The listing builds one solid part. Answer for the finished solid, in the listing's coordinates (mm). A direction names the side the tool comes from. Coordinates: 2 decimals unless noted, no trailing zeros. Order: outer loops, then holes, each group sorted by start corner. A loop starts at its lowest first (then second) coordinate and runs counter-clockwise, first axis right, second up. Notation, with made-up numbers: (43, 4) -> (91, 4) arc R22 ccw to (91, 16) -> close; hole circle Ø7 at (-20, 45). An arc over 180 degrees is marked (long way). Return JSON: item names as keys, results as strings.
```python
from build123d import *

# Parameters (mm, degrees)
REVOLVE_OF_12_NOM_W          = 584.2
REVOLVE_OF_12_NOM_H          = 20.193
F_6_NOM_OD_EXTRUDE_REACH     = 570.325
SKETCH2_R                    = 84.1375
F_6_NOM_ID_EXTRUDE_CUT_REACH = 570.325
F_6_NOM_ID_EXTRUDE_R         = 73.6473


with BuildPart() as part:
    # Revolve of 12 NOM → Revolve12 NOM (revolve)
    with BuildSketch(Plane.XY):
        with Locations((0, 151.8285)):
            Rectangle(REVOLVE_OF_12_NOM_W, REVOLVE_OF_12_NOM_H)
    revolve(axis=Axis((0, 0, 0), (1, 0, 0)))

    # Sketch2 → 6 NOM OD Extrude (add, up to next)
    with BuildSketch(Plane(origin=(0, 406.4, 0), x_dir=(1, 0, 0), z_dir=(0, 1, 0)), mode=Mode.PRIVATE) as f_6_nom_od_extrude_sk1:
        Circle(SKETCH2_R)
    f_6_nom_od_extrude_tool1 = extrude(f_6_nom_od_extrude_sk1.sketch, amount=-F_6_NOM_OD_EXTRUDE_REACH, mode=Mode.PRIVATE) - part.part
    add(f_6_nom_od_extrude_tool1.solids().sort_by_distance((0, 406.4, 0))[0])

    # 6 NOM ID Extrude → 6 NOM ID Extrude Cut (cut, up to next)
    with BuildSketch(Plane(origin=(0, 406.4, 0), x_dir=(1, 0, 0), z_dir=(0, 1, 0)), mode=Mode.PRIVATE) as f_6_nom_id_extrude_cut_sk1:
        Circle(F_6_NOM_ID_EXTRUDE_R)
    f_6_nom_id_extrude_cut_tool1 = extrude(f_6_nom_id_extrude_cut_sk1.sketch, amount=-F_6_NOM_ID_EXTRUDE_CUT_REACH, mode=Mode.PRIVATE) & part.part
    add(f_6_nom_id_extrude_cut_tool1.solids().sort_by_distance((0, 406.4, 0))[0], mode=Mode.SUBTRACT)


solid = part.part
```
Item 1: Find the intervals of material crossed by probe 1 along Z at (x, y) = (76, 0) (3 decimals); probe 2 along Z at (x, y) = (-24, -5.5); probe 3 along X at (y, z) = (331, 0), in increasing order.
Answer list:
{"probe 1": "-161.925 to -141.732, 141.732 to 161.925", "probe 2": "-161.83 to -141.63, 141.63 to 161.83", "probe 3": "-84.14 to -73.65, 73.65 to 84.14"}
Item 2: Flat-ended cylindrical pins translate along their axes: pin 1 (5 mm diameter, centred on y = 312, z = -50, fed in from -X); pin 2 (10 mm diameter, centred on x = 151.5, z = 116, fed in from -Y); pin 3 (6 mm diameter, centred on x = 21.5, y = 273.5, fed in from +Z). Find the tip coordinate at first contact, or state that the pin passes through.
Answer list:
{"pin 1": "x = -69.45", "pin 2": "y = -117.89", "pin 3": "z = 82.08"}
Item 3: The part is cut by section B-B on z = 0. Determine the outline of the cut face in (x, y) (1 decimal), plus the area to 3 significant figures.
Answer list:
{"outline": "(-292.1, -161.9) -> (292.1, -161.9) -> (292.1, -141.7) -> (-292.1, -141.7) -> close; (-292.1, 141.7) -> (-73.6, 141.7) -> (-73.6, 406.4) -> (-84.1, 406.4) -> (-84.1, 161.9) -> (-292.1, 161.9) -> close; (73.6, 141.7) -> (292.1, 141.7) -> (292.1, 161.9) -> (84.1, 161.9) -> (84.1, 406.4) -> (73.6, 406.4) -> close", "area": "25,700 mm2"}
Item 4: Which of the six approach directions +Z, -Z, +X, -X, +Y, -Y give full straight-line access (tool end or side, diameter ignored) to faces 1 (the cylindrical face through (-15.965, 265.745, 71.896)), 2 (the flat face through (-292.1, 1, -143))?
Answer list:
{"face 1": "+Y", "face 2": "+Z, -Z, -X, +Y, -Y"}
Item 5: The part is cut by section A-A on y = 0. Determine the outline of the cut face in (x, z) (3 decimals).
Answer list:
{"outline": "(-292.1, -161.925) -> (292.1, -161.925) -> (292.1, -141.732) -> (-292.1, -141.732) -> close; (-292.1, 141.732) -> (292.1, 141.732) -> (292.1, 161.925) -> (-292.1, 161.925) -> close"}
Item 6: The part is cut by section D-D on z = 101.5. Determine the outline of the cut face in (x, y).
Answer list:
{"outline": "(-292.1, -126.16) -> (292.1, -126.16) -> (292.1, -98.92) -> (-292.1, -98.92) -> close; (-292.1, 98.92) -> (292.1, 98.92) -> (292.1, 126.16) -> (-292.1, 126.16) -> close"}
Item 7: Determine the mould class of faces 3 (the flat face through (0, 406.4, 74)), 4 (the cylindrical face through (-84.056, 274.251, -3.699)), 5 (the cylindrical face through (4.089, -141.595, 6.232)) for opening direction Z: pulls with the +Z half, pulls with the -Z half, needs draft (parallel to the pull), parting line crosses it, or undercut.
Answer list:
{"face 3": "needs draft", "face 4": "parting line crosses it", "face 5": "undercut"}
